Check sheet for the drawn part. Datum: minimum x, y, z corner. Units: mm. A direction names the side the tool comes from. Give positions to 0.01 mm unless a question says otherwise; leave off trailing zeros. Loops run counter-clockwise (first coordinate to the right, second up) from the corner with the lowest first, then second, coordinate; pieces in that order, holes last.
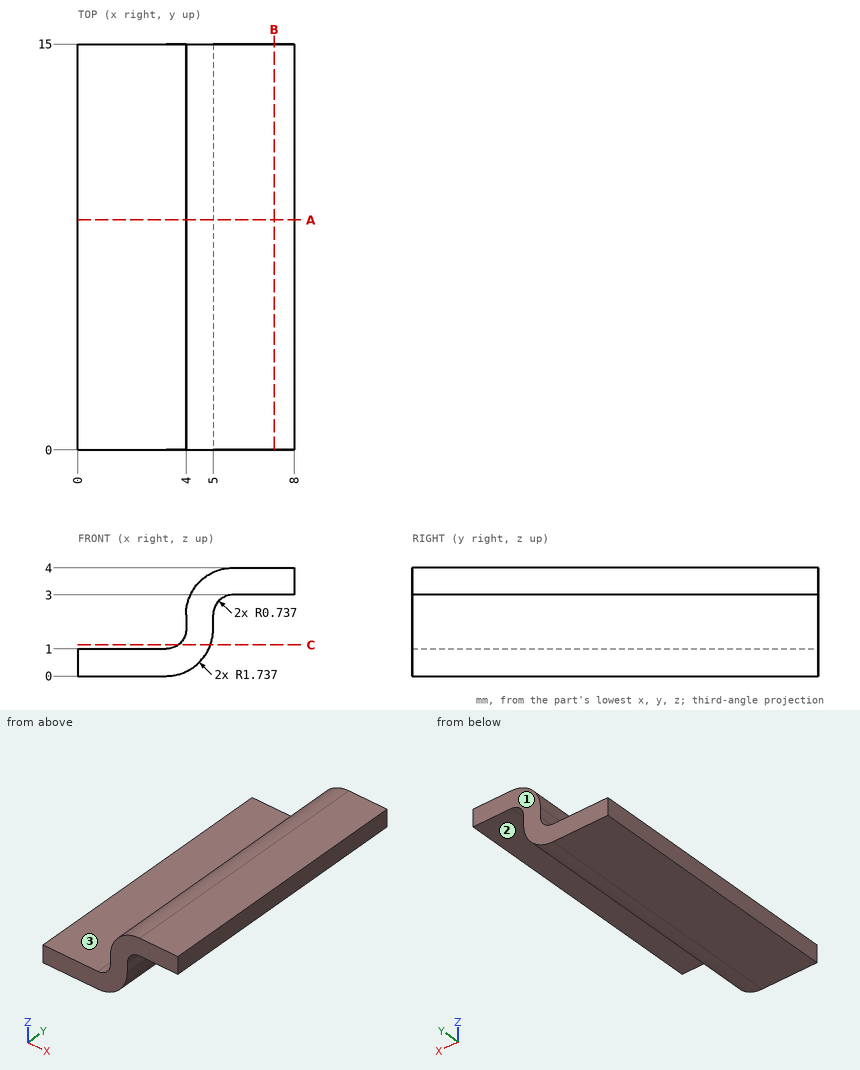
1) Sectioned sample at A-A on y = 8.5. Enter the section's corners in (x, z).
2) Sectioned sample at B-B on x = 7.25. Enter the section's corners in (y, z), plus the area to 3 significant figures.
3) Tool access check on the marked faces 1, 2 and 3. Record the directions out of +Z, -Z, +X, -X, +Y, -Y that give a thin tool (end or side, any length) a straight path to the whole face; none if there is none.
4) Depth check by flat-ended pin: P1, Ø3.5, axis at x = 2, y = 11, coming from the +Z side (1 decimal); P2, Ø1.1, axis at x = 7, y = 5.5, coming from the -Z side; P3, Ø3, axis at x = 5, y = 5.5, coming from the -Z side. Enter the tip coordinate at first touch or a pass-through.
5) Scan lines: line 1 along Z through (x, y) = (3, 10.25); line 2 along Z through (x, y) = (6.75, 11); line 3 along X through (y, z) = (4, 2.2). Record each from-to range of solid material in increasing order.
6) Sectioned sample at C-C on z = 1.15. Enter the section's corners in (x, y).
Determined:
1. outline: (0, 0) - (3.26, 0) arc R1.74 ccw to (5, 1.74) - (5, 2.26) arc R0.74 cw to (5.74, 3) - (8, 3) - (8, 4) - (5.74, 4) arc R1.74 ccw to (4, 2.26) - (4, 1.74) arc R0.74 cw to (3.26, 1) - (0, 1) - close
2. outline: (0, 3) - (15, 3) - (15, 4) - (0, 4) - close
2. area: 15.0 mm2
3. face 1: +Z, -Z, +X, -X, +Y
3. face 2: -Z, +X, +Y, -Y
3. face 3: +Z, -X, +Y, -Y
4. P1: stops at z = 1.2
4. P2: stops at z = 3
4. P3: stops at z = 0.02
5. line 1: z = 0 to 1
5. line 2: z = 3 to 4
5. line 3: x = 4 to 5
6. outline: (3.71, 0) - (4.9, 0) - (4.9, 15) - (3.71, 15) - close
